from build123d import *

# Parameters (mm, degrees)
BOX_W        = 10
BOX_H        = 10
BOX_DEPTH    = 30
BOX001_W     = 10
BOX001_H     = 10
BOX001_DEPTH = 20
BOX002_W     = 10
BOX002_H     = 10
BOX002_DEPTH = 20
BOX003_W     = 10
BOX003_H     = 10
BOX003_DEPTH = 10
BOX004_W     = 10
BOX004_H     = 10
BOX004_DEPTH = 10


with BuildPart() as nivell1_cub1:
    # Box → Box (new body)
    with BuildSketch(Plane.XY):
        with Locations((5, 5)):
            Rectangle(BOX_W, BOX_H)
    extrude(amount=BOX_DEPTH)


with BuildPart() as nivell1_cub2:
    # Box001 → Box001 (new body)
    with BuildSketch(Plane(origin=(10, 0, 0), x_dir=(1, 0, 0), z_dir=(0, 0, 1))):
        with Locations((5, 5)):
            Rectangle(BOX001_W, BOX001_H)
    extrude(amount=BOX001_DEPTH)


with BuildPart() as nivell1_cub3:
    # Box002 → Box002 (new body)
    with BuildSketch(Plane(origin=(0, 10, 0), x_dir=(1, 0, 0), z_dir=(0, 0, 1))):
        with Locations((5, 5)):
            Rectangle(BOX002_W, BOX002_H)
    extrude(amount=BOX002_DEPTH)


with BuildPart() as nivell1_cub4:
    # Box003 → Box003 (new body)
    with BuildSketch(Plane(origin=(20, 0, 0), x_dir=(1, 0, 0), z_dir=(0, 0, 1))):
        with Locations((5, 5)):
            Rectangle(BOX003_W, BOX003_H)
    extrude(amount=BOX003_DEPTH)


with BuildPart() as fusion:
    # Box004 → Box004 (new body)
    with BuildSketch(Plane(origin=(0, 20, 0), x_dir=(1, 0, 0), z_dir=(0, 0, 1))):
        with Locations((5, 5)):
            Rectangle(BOX004_W, BOX004_H)
    extrude(amount=BOX004_DEPTH)

    # Fusion: union nivell1_cub1, nivell1_cub2, nivell1_cub3, nivell1_cub4
    add(nivell1_cub1.part)
    add(nivell1_cub2.part)
    add(nivell1_cub3.part)
    add(nivell1_cub4.part)


solid = fusion.part
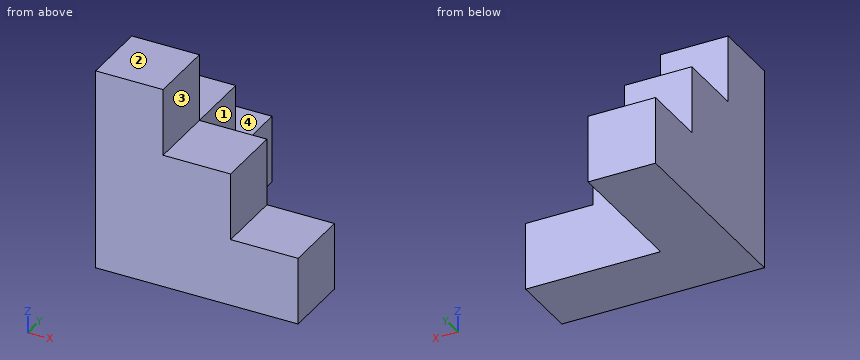
Input: part model. Units: mm. Frame: model coordinates. Face numbers are marked on the shaded views. A direction names the side the tool comes from. Give positions to 0.01 mm unless a question says otherwise; leave off trailing zeros. Write each loop counter-clockwise with the first axis right and the second up, starting at its lowest first coordinate (ties: lowest second). Pieces come first, ordered by that corner, then holes. Notation, with made-up numbers: M -39,62.25 L 16,62.25 A25 cw 16,76.25 Z; hole C 64,2.25 d2. An arc over 180 degrees is marked long. Use one line per item in the form item = value.
1. First-contact query: P1, Ø8, axis at x = 17.5, y = 2.5, coming from the +Z side; P2, Ø12, axis at x = 24, z = 17.5, coming from the +Y side; P3, Ø3, axis at x = 27, y = 4.5, coming from the +Z side. Flat tips, straight axial feed; report the tip coordinate or a pass-through.
Outcome:
P1 = 20
P2 = 10
P3 = 10
2. Ray query, L1, parallel to Y at x = 6.25, z = 14; L2, parallel to Y at x = 18.25, z = 7.75. Return the intervals inside material, ascending.
Outcome:
L1 = 0 to 20
L2 = 0 to 10
3. Cut plane A-A on z = 2.25. Return loops of the section in (x, y), and give its area (3 significant figures).
Outcome:
outline = M 0,0 L 30,0 L 30,10 L 10,10 L 10,30 L 0,30 Z
area = 500 mm²
4. Reachability of the marked faces 1, 2, 3 and 4 from +Z, -Z, +X, -X, +Y, -Y: full face, straight path, thin tool, end or side. Return the list, or none.
Outcome:
face_1 = +Z, -Z, +X, +Y
face_2 = +Z, +X, -X, +Y, -Y
face_3 = +Z, +X, +Y, -Y
face_4 = +Z, +X, -X, +Y
5. Cut plane D-D on x = 16.25. Return loops of the section in (y, z).
Outcome:
outline = M 0,0 L 10,0 L 10,20 L 0,20 Z
6. Cut plane B-B on y = 7. Return loops of the section in (x, z), and give its area (3 significant figures).
Outcome:
outline = M 0,0 L 30,0 L 30,10 L 20,10 L 20,20 L 10,20 L 10,30 L 0,30 Z
area = 600 mm²
